Work out the finished part from the listing and answer in its coordinate system (mm). Face numbers are marked on the shaded views. A direction names the side the tool comes from. Round coordinates to 2 decimals unless told otherwise and drop trailing zeros. Write each loop counter-clockwise with the first axis right and the second up, starting at its lowest first coordinate (ties: lowest second). Pieces come first, ordered by that corner, then holes.
1. Find section C-C (x = 32.5). Write down the section's boundary in (y, z).
2. A tool of negligible diameter and unlimited length cuts with its end or side. For the marked faces 1, 2 and 3, from which of +Z, -Z, +X, -X, +Y, -Y can it reach the whole face along a straight path? Write none if from no direction.
3. Determine the mould class of the marked faces 4, 5 and 6 for opening direction X: pulls with the +X half, pulls with the -X half, needs draft (parallel to the pull), parting line crosses it, or undercut.
4. Flat-ended cylindrical pins translate along their axes: pin 1 Ø1.8 at (x, y) = (2, 12.5) entering from +Z; pin 2 Ø10 at (y, z) = (25.5, 42.5) entering from -X; pin 3 Ø10 at (x, z) = (60, 40) entering from -Y; pin 4 Ø3 at (x, z) = (26.5, 33) entering from +Y. Find the tip coordinate at first contact, or state that the pin passes through.
5. Find section A-A (z = 19.05). Count the separate pieces of the cut face and the enclosed holes in it, and give its area (3 significant figures).
6. Straight lines are drawn through the part: probe 1 along X at (y, z) = (35, 44.45); probe 2 along Z at (x, y) = (76.29, 35.9); probe 3 along X at (y, z) = (-11, 47.5). For each, find the intervals that lie inside material, in ascending order.
7. Find section D-D (z = 50.5). Write down the section's boundary in (x, y).
8. Find section B-B (x = 76.29). Write down the section's boundary in (y, z).
```python
from build123d import *

# Parameters (mm, degrees)
SKETCH1_W           = 125
SKETCH1_H           = 76.2
BOSS_EXTRUDE1_DEPTH = 3
SKETCH2_W           = 5
SKETCH2_H           = 76.2
BOSS_EXTRUDE2_DEPTH = 55
SKETCH4_W           = 58
SKETCH4_H           = 5
BOSS_EXTRUDE4_DEPTH = 21.59
SKETCH5_W           = 58
SKETCH5_H           = 5
BOSS_EXTRUDE5_DEPTH = 21.59
SKETCH6_W           = 168.18
SKETCH6_H           = 25.4
BOSS_EXTRUDE6_DEPTH = 3
CHAMFER1_SIZE       = 28
SKETCH7_W           = 89.6
SKETCH7_H           = 26
CUT_EXTRUDE1_DEPTH  = 2
SKETCH9_W           = 115
SKETCH9_H           = 3
BOSS_EXTRUDE7_DEPTH = 55
CHAMFER2_SIZE       = 4
CHAMFER3_SIZE       = 5
CUT_EXTRUDE2_START  = -0.6
CUT_EXTRUDE2_DEPTH  = 0.6
SKETCH11_R          = 1.75
CUT_EXTRUDE3_DEPTH  = 5
SKETCH12_R          = 1.75
CUT_EXTRUDE4_DEPTH  = 5
FILLET1_R           = 1
CHAMFER4_SIZE       = 1.5


# Read off the part's stored shape, not the designer's step: Cut-Extrude2
with BuildPart() as part:
    # Sketch1 → Boss-Extrude1 (new body)
    with BuildSketch(Plane.XY):
        Rectangle(SKETCH1_W, SKETCH1_H)
    extrude(amount=BOSS_EXTRUDE1_DEPTH)

    # Sketch2 → Boss-Extrude2 (add)
    with BuildSketch(Plane.XY.offset(3)):
        with Locations((-60, 0)):
            Rectangle(SKETCH2_W, SKETCH2_H)
        with Locations((60, 0)):
            Rectangle(SKETCH2_W, SKETCH2_H)
    extrude(amount=BOSS_EXTRUDE2_DEPTH)

    # Sketch4 → Boss-Extrude4 (add)
    with BuildSketch(Plane.ZY.offset(62.5)):
        with Locations((29, 35.6)):
            Rectangle(SKETCH4_W, SKETCH4_H)
    extrude(amount=BOSS_EXTRUDE4_DEPTH)

    # Sketch5 → Boss-Extrude5 (add)
    with BuildSketch(Plane(origin=(62.5, 0, 0), x_dir=(0, 0, -1), z_dir=(1, 0, 0))):
        with Locations((-29, 35.6)):
            Rectangle(SKETCH5_W, SKETCH5_H)
    extrude(amount=BOSS_EXTRUDE5_DEPTH)

    # Sketch6 → Boss-Extrude6 (add)
    with BuildSketch(Plane(origin=(0, 0, 0), x_dir=(-1, 0, 0), z_dir=(0, 0, -1))):
        with Locations((0, 50.8)):
            Rectangle(SKETCH6_W, SKETCH6_H)
    extrude(amount=-BOSS_EXTRUDE6_DEPTH)

    # Chamfer1
    chamfer1_edges = [part.edges().sort_by_distance(p)[0] for p in [
        (-84.09, 63.5, 1.5),
        (84.09, 63.5, 1.5),
    ]]
    chamfer(chamfer1_edges, length=CHAMFER1_SIZE)

    # Sketch7 → Cut-Extrude1 (cut)
    with BuildSketch(Plane.XY.offset(3)):
        with Locations((0, -9.4)):
            Rectangle(SKETCH7_W, SKETCH7_H)
        with Locations((0, 36.6)):
            Rectangle(SKETCH7_W, SKETCH7_H)
    extrude(amount=-CUT_EXTRUDE1_DEPTH, mode=Mode.SUBTRACT)

    # Sketch9 → Boss-Extrude7 (add)
    with BuildSketch(Plane.XY.offset(3)):
        with Locations((0, -36.6)):
            Rectangle(SKETCH9_W, SKETCH9_H)
    extrude(amount=BOSS_EXTRUDE7_DEPTH)

    # Chamfer2
    chamfer2_edges = [part.edges().sort_by_distance(p)[0] for p in [
        (-57.5, -35.1, 30.5),
        (57.5, -35.1, 30.5),
    ]]
    chamfer(chamfer2_edges, length=CHAMFER2_SIZE)

    # Chamfer3
    chamfer3_edges = [part.edges().sort_by_distance(p)[0] for p in [
        (62.5, -38.1, 29),
        (-62.5, -38.1, 29),
    ]]
    chamfer(chamfer3_edges, length=CHAMFER3_SIZE)

    # Cut-Extrude2 outline → Cut-Extrude2 (cut)
    # profile 1 of 4: a face of its own
    with BuildSketch(Plane.XY.offset(3).offset(CUT_EXTRUDE2_START)):
        with BuildLine():
            Line((-12.843793417, 16.784775128), (-13.918894641, 13.722312614))
            add(Edge.make_bspline(
                [(-13.918894641, 13.722312614), (-13.950745906, 13.608646354), (-13.97919001, 13.483685694), (-14.011317489, 13.235305925), (-14.01541758, 13.110841548), (-13.989547543, 12.867284383), (-13.959604678, 12.747961158), (-13.857332343, 12.519974586), (-13.78490702, 12.411398187), (-13.592313629, 12.212018271), (-13.472083062, 12.121314997), (-13.184369222, 11.962818623), (-13.016909084, 11.895027419), (-12.454211206, 11.728033285), (-11.997806272, 11.664794493), (-11.025815686, 11.62704002), (-10.511530183, 11.651603075), (-9.78258436, 11.770518687), (-9.546683753, 11.824200176), (-9.102156978, 11.962599668), (-8.89364967, 12.047436893), (-8.514064046, 12.246658938), (-8.343153207, 12.361026326), (-8.04132547, 12.611058926), (-7.910418089, 12.746448479), (-7.679883041, 13.0275306), (-7.579636344, 13.172799488), (-7.44297026, 13.39668043), (-7.39971151, 13.472431032), (-7.318663078, 13.627460279), (-7.280772846, 13.706786212), (-7.248185858, 13.788667895)],
                knots=[0, 0, 0, 0, 0.0625, 0.0625, 0.125, 0.125, 0.1875, 0.1875, 0.25, 0.25, 0.3125, 0.3125, 0.375, 0.375, 0.5, 0.5, 0.625, 0.625, 0.6875, 0.6875, 0.75, 0.75, 0.8125, 0.8125, 0.875, 0.875, 0.9375, 0.9375, 0.96875, 0.96875, 1, 1, 1, 1], degree=3))
            Line((-7.248185858, 13.788667895), (-6.196379448, 16.784775128))
            Line((-6.196379448, 16.784775128), (-7.771512854, 16.784775171))
            Line((-7.771512854, 16.784775171), (-8.779640442, 13.913087848))
            add(Edge.make_bspline(
                [(-8.779640442, 13.913087848), (-8.801212863, 13.867686768), (-8.828630281, 13.811426743), (-8.890437912, 13.684919137), (-8.925723343, 13.615289873), (-9.014867696, 13.477778317), (-9.069034752, 13.410065742), (-9.20356673, 13.286811644), (-9.283951715, 13.231246188), (-9.470687062, 13.136081945), (-9.576947425, 13.096402347), (-9.809000897, 13.032201026), (-9.934689567, 13.00760449), (-10.326953956, 12.952228061), (-10.607716868, 12.939250309), (-11.138236784, 12.940792557), (-11.387946526, 12.95495502), (-11.815776289, 13.010911905), (-11.994686961, 13.05312605), (-12.19022456, 13.154353945), (-12.243244201, 13.194586759), (-12.322270156, 13.289978248), (-12.348136332, 13.345299657), (-12.373130151, 13.46826163), (-12.371956966, 13.5361378), (-12.35254935, 13.67085438), (-12.333771283, 13.737944141), (-12.322165603, 13.788667937)],
                knots=[0, 0, 0, 0, 0.0625, 0.0625, 0.125, 0.125, 0.1875, 0.1875, 0.25, 0.25, 0.3125, 0.3125, 0.375, 0.375, 0.5, 0.5, 0.625, 0.625, 0.75, 0.75, 0.8125, 0.8125, 0.875, 0.875, 0.9375, 0.9375, 1, 1, 1, 1], degree=3))
            Line((-12.322165603, 13.788667937), (-11.2703582, 16.784775128))
            Line((-11.2703582, 16.784775128), (-12.843793417, 16.784775128))
        make_face()
    # profile 2 of 4: a face of its own
    with BuildSketch(Plane.XY.offset(3).offset(CUT_EXTRUDE2_START)):
        Polygon((14.082145905, 15.466432145), (14.547318434, 16.784775128), (8.481425261, 16.784775128), (8.015662645, 15.45803385), (10.386127447, 15.45803385), (9.075451111, 11.743439605), (10.661733364, 11.743439605), (11.975372051, 15.466432145), align=None)
    # profile 3 of 4: a face of its own
    with BuildSketch(Plane.XY.offset(3).offset(CUT_EXTRUDE2_START)):
        Polygon((0.359928822, 15.45803385), (0.825593089, 16.784775128), (-5.237786258, 16.784775128), (-5.705919648, 15.45803385), (-3.328357423, 15.45803385), (-4.639000977, 11.723834147), (-3.059652234, 11.723834147), (-1.74900868, 15.45803385), align=None)
    # profile 4 of 4: a face of its own
    with BuildSketch(Plane.XY.offset(3).offset(CUT_EXTRUDE2_START)):
        Polygon((7.732615088, 18.009820452), (8.67993853, 22.298690548), (4.451236342, 18.010625114), (-13.617285872, 18.010625114), (-13.760696138, 17.631800344), (4.083976363, 17.631800344), (-2.561139847, 10.89339914), (-16.036862666, 10.89339914), (-16.175076152, 10.505618026), (-2.943552817, 10.505618026), (-8.264964605, 5.10950355), (-0.819885517, 10.505618026), (5.569839691, 10.505618026), (5.813932632, 9.32327198), (6.07620201, 10.510665049), (13.482070183, 10.510665049), (13.624063348, 10.89339914), (6.160742258, 10.89339914), (7.649117922, 17.631800344), (15.972876762, 17.631800344), (16.113123511, 18.009820452), align=None)
        Polygon((-0.283933962, 10.894070437), (4.780674194, 14.564845582), (5.489286994, 10.894070437), align=None, mode=Mode.SUBTRACT)
        Polygon((5.863139247, 17.323666682), (5.364033793, 14.945937564), (5.179256414, 15.9244998), (2.885975157, 14.289472868), align=None, mode=Mode.SUBTRACT)
    extrude(amount=CUT_EXTRUDE2_DEPTH, mode=Mode.SUBTRACT)

    # Sketch11 → Cut-Extrude3 (cut)
    with BuildSketch(Plane(origin=(0, 38.1, 0), x_dir=(1, 0, 0), z_dir=(0, 1, 0))):
        with Locations(Location((-76.11, -19.05, 0), (0, 0, 270))):
            Circle(SKETCH11_R)
        with Locations(Location((76.29, -19.05, 0), (0, 0, 270))):
            Circle(SKETCH11_R)
    extrude(amount=-CUT_EXTRUDE3_DEPTH, mode=Mode.SUBTRACT)

    # Sketch12 → Cut-Extrude4 (cut)
    with BuildSketch(Plane(origin=(0, 38.1, 0), x_dir=(1, 0, 0), z_dir=(0, 1, 0))):
        with Locations(Location((-76.11, -44.45, 0), (0, 0, 270))):
            Circle(SKETCH12_R)
        with Locations(Location((76.29, -44.45, 0), (0, 0, 270))):
            Circle(SKETCH12_R)
    extrude(amount=-CUT_EXTRUDE4_DEPTH, mode=Mode.SUBTRACT)

    # Fillet1
    fillet1_edges = [part.edges().sort_by_distance(p)[0] for p in [
        (-62.5, 33.1, 29),
        (62.5, 33.1, 29),
    ]]
    fillet(fillet1_edges, radius=FILLET1_R)

    # Chamfer4
    chamfer4_edges = [part.edges().sort_by_distance(p)[0] for p in [
        (-57.5, 38.1, 30.5),
        (57.5, 38.1, 30.5),
    ]]
    chamfer(chamfer4_edges, length=CHAMFER4_SIZE)


solid = part.part
```
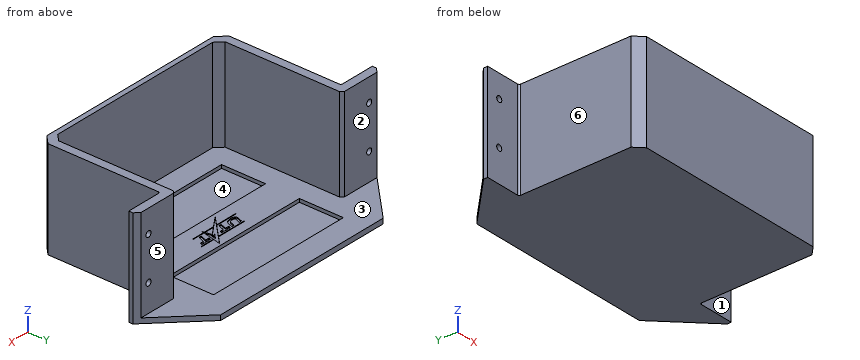
Worked answers:
1. outline: (-38.1, 0) - (63.5, 0) - (63.5, 3) - (49.6, 3) - (49.6, 1) - (23.6, 1) - (23.6, 3) - (3.6, 3) - (3.6, 1) - (-22.4, 1) - (-22.4, 3) - (-35.1, 3) - (-35.1, 58) - (-38.1, 58) - close
2. face 1: +Z, -Z, +X, -Y
2. face 2: +Z, +X, -X, +Y
2. face 3: +Z, +Y
3. face 4: undercut
3. face 5: needs draft
3. face 6: pulls with the -X half
4. pin 1: stops at z = 3
4. pin 2: stops at x = -62.5
4. pin 3: stops at y = -38.1
4. pin 4: stops at y = -35.1
5. separate pieces: 3
5. enclosed holes: 0
5. area: 1,270 mm2
6. probe 1: x = -84.09 to -77.86, -74.36 to -57.5, 57.5 to 74.54, 78.04 to 84.09
6. probe 2: z = 0 to 17.3, 20.8 to 42.7, 46.2 to 58
6. probe 3: x = -62.5 to -57.5, 57.5 to 62.5
7. outline: (-84.09, 33.1) - (-63.5, 33.1) arc R1 cw to (-62.5, 32.1) - (-62.5, -33.1) - (-57.5, -38.1) - (57.5, -38.1) - (62.5, -33.1) - (62.5, 32.1) arc R1 cw to (63.5, 33.1) - (84.09, 33.1) - (84.09, 35.5) - (81.49, 38.1) - (59, 38.1) - (57.5, 36.6) - (57.5, -31.1) - (53.5, -35.1) - (-53.5, -35.1) - (-57.5, -31.1) - (-57.5, 36.6) - (-59, 38.1) - (-81.49, 38.1) - (-84.09, 35.5) - close
8. outline: (33.1, 0) - (43.3, 0) - (43.3, 3) - (38.1, 3) - (38.1, 17.3) - (33.1, 17.3) - close; (33.1, 20.8) - (38.1, 20.8) - (38.1, 42.7) - (33.1, 42.7) - close; (33.1, 46.2) - (38.1, 46.2) - (38.1, 58) - (33.1, 58) - close
